from build123d import *

# Parameters (mm, degrees)
EXTRUDE_1_DEPTH          = 20
SKETCH_2_R               = 1.1
CUT_EXTRUDE_2_DEPTH      = 26.709920264
CUT_EXTRUDE_3_REACH      = 29.731
SKETCH_3_W               = 30
SKETCH_3_H               = 15.1
FILLET_1_R               = 3
SKETCH_6_W               = 30.918408881
SKETCH_6_H               = 20
SKETCH_6_W_2             = 27.918408881
SKETCH_6_H_2             = 17
EXTRUDE_2_DEPTH          = 2.5
CUT_EXTRUDE_4_DEPTH      = 25.9500604
CUT_EXTRUDE_4_DEPTH_BACK = 25.9500604


with BuildPart() as part:
    # 草图1 → 凸台-拉伸1 (new body)
    with BuildSketch(Plane(origin=(0, 0, 0), x_dir=(1, 0, 0), z_dir=(0, 1, 0))):
        Polygon((-15, -6), (15, 1.479840085), (15, 6), (-15, 6), align=None)
    extrude(amount=EXTRUDE_1_DEPTH)

    # 草图2 → 切除-拉伸2 (cut, through all)
    with BuildSketch(Plane(origin=(0, 20, 0), x_dir=(1, 0, 0), z_dir=(0, 1, 0))):
        with Locations(Location((-12.5, 3, 0), (0, 0, 270))):
            Circle(SKETCH_2_R)
        with Locations(Location((-7.537269242, 3.609346717, 0), (0, 0, 270))):
            Circle(SKETCH_2_R)
        with Locations(Location((-2.574538484, 4.218693434, 0), (0, 0, 270))):
            Circle(SKETCH_2_R)
    extrude(amount=-CUT_EXTRUDE_2_DEPTH, mode=Mode.SUBTRACT)

    # 切除-拉伸3: up to this plane
    cut_extrude_3_end = Plane(origin=(0.167638791, 0, 0.672362468), z_dir=(0.24192189559966876, 0, 0.9702957262759963))
    # 草图3 → 切除-拉伸3 (cut, up to the surface)
    with BuildSketch(Plane(origin=(0, 0, -6), x_dir=(-1, 0, 0), z_dir=(0, 0, -1)), mode=Mode.PRIVATE) as cut_extrude_3_sk1:
        with Locations((0, 10)):
            Rectangle(SKETCH_3_W, SKETCH_3_H)
    cut_extrude_3_tool1 = split(extrude(cut_extrude_3_sk1.sketch, amount=-CUT_EXTRUDE_3_REACH, mode=Mode.PRIVATE), bisect_by=cut_extrude_3_end, keep=Keep.BOTH, mode=Mode.PRIVATE)
    add(cut_extrude_3_tool1.solids().sort_by_distance((0, 10, -6))[0], mode=Mode.SUBTRACT)

    # 圆角1
    fillet_1_edges = [part.edges().sort_by_distance(p)[0] for p in [
        (-15, 1.225, -6),
        (-15, 18.775, -6),
    ]]
    fillet(fillet_1_edges, radius=FILLET_1_R)

    # 草图6 → 凸台-拉伸2 (add)
    with BuildSketch(Plane(origin=(0.530521635, 0, 2.127806058), x_dir=(0.9702957262759964, 0, -0.2419218955996687), z_dir=(0.2419218955996687, 0, 0.9702957262759964))):
        with Locations((-0.546762828, 10)):
            Rectangle(SKETCH_6_W, SKETCH_6_H)
        with Locations((-0.546762828, 10)):
            Rectangle(SKETCH_6_W_2, SKETCH_6_H_2, mode=Mode.SUBTRACT)
    extrude(amount=EXTRUDE_2_DEPTH)

    # 草图7 → 切除-拉伸4 (cut, two sides: drawn at the far end of the back side and taken through both)
    with BuildSketch(Plane(origin=(0, 2.45, 0), x_dir=(1, 0, 0), z_dir=(0, 1, 0)).offset(-CUT_EXTRUDE_4_DEPTH_BACK)):
        Polygon((15, 3.025760529), (4, 6), (15, 6), align=None)
    extrude(amount=CUT_EXTRUDE_4_DEPTH + CUT_EXTRUDE_4_DEPTH_BACK, mode=Mode.SUBTRACT)


solid = part.part
The listing builds one solid part. Answer for the finished solid, in the listing's coordinates (mm). A direction names the side the tool comes from. Coordinates: 2 decimals unless noted, no trailing zeros. Write each loop counter-clockwise with the first axis right and the second up, starting at its lowest first coordinate (ties: lowest second). Pieces come first, ordered by that corner, then holes. Notation, with made-up numbers: M 54,46 L 64,46 A20 cw 64,83 Z; hole C 83,28 d2. An arc over 180 degrees is marked long. Put each result on its own line as item: value. Start each with the question number.
1. A cutting plane is placed at B-B on x = -12.5. Write down the section's boundary in (y, z).
2. For a pull along Y with two mould halves and no side action, classify faces 1 (the flat face through (-0.21, 10.106, 0.767)), 2 (the flat face through (-1, 20, 0)), 3 (the flat face through (9.58, 1.21, -4.49)) as pulls with the +Y half, pulls with the -Y half, needs draft (parallel to the pull), parting line crosses it, or undercut.
3. Which of the six approach directions +Z, -Z, +X, -X, +Y, -Y give full straight-line access (tool end or side, diameter ignored) to faces 4 (the flat face through (15, 10, -2)), 5 (the flat face through (-4, 1, -6)), 6 (the flat face through (-3, 17.55, -2)), 7 (the cylindrical face through (-14.14, 1.24, -5.1)), 8 (the flat face through (13.843, 9.881, 0.079))?
4. A cutting plane is placed at D-D on x = 8. Write down the section's boundary in (y, z).
5. Consider line 1 (Y direction, x = 10.5, z = 0); line 2 (Y direction, x = -3, z = 0); line 3 (X direction, y = 18.4, z = -3). Determine where each line is inside the solid, lowest interval first. Write a range as from..to.
6. A cutting plane is placed at A-A on y = 15. Write down the section's boundary in (x, z).
7. Flat-ended cylindrical pins translate along their axes: P1, Ø1, axis at x = 0, y = 3.5, coming from the -Z side; P2, Ø10, axis at x = 6, y = 14.5, coming from the +Z side; P3, Ø2, axis at x = -12.5, z = -3, coming from the +Y side; P4, Ø6, axis at y = 10, z = -3, coming from the +X side. Find the tip coordinate at first contact, or state that the pin passes through.
8. A cutting plane is placed at C-C on z = 3.25. Write down the section's boundary in (x, y).
Resolved:
1. outline: M 0,-5.96 L 2.45,-5.96 L 2.45,-4.1 L 0,-4.1 Z; M 0,-1.9 L 2.45,-1.9 L 2.45,3.83 L 17.55,3.83 L 17.55,-1.9 L 20,-1.9 L 20,7.95 L 18.5,7.95 L 18.5,5.38 L 1.5,5.38 L 1.5,7.95 L 0,7.95 Z; M 17.55,-5.96 L 20,-5.96 L 20,-4.1 L 17.55,-4.1 Z
2. face 1: undercut
2. face 2: pulls with the +Y half
2. face 3: needs draft
3. face 4: -Z, +X, +Y, -Y
3. face 5: -Z, +X, -X, +Y, -Y
3. face 6: -Z, -X
3. face 7: -Z, -X, +Y, -Y
3. face 8: +Z
4. outline: M 0,-4.92 L 2.45,-4.92 L 2.45,-1.28 L 17.55,-1.28 L 17.55,-4.92 L 20,-4.92 L 20,2.84 L 18.5,2.84 L 18.5,0.27 L 1.5,0.27 L 1.5,2.84 L 0,2.84 Z
5. line 1: y = 0..1.5, 18.5..20
5. line 2: y = 0..2.45, 17.55..20
5. line 3: x = -15..-13.6, -11.4..-8.45, -6.62..15
6. outline: M -15,4.45 L 15,-3.03 L 15,-1.48 L 15.6,0.95 L 14.15,1.31 L 13.54,-1.12 L -13.54,5.64 L -12.94,8.06 L -14.4,8.43 L -15,6 Z
7. P1: stops at z = 0.59
7. P2: stops at z = 4.09
7. P3: passes through
7. P4: stops at x = 15.37
8. outline: M -15,0 L 6.36,0 L 6.36,1.5 L -3.97,1.5 L -3.97,18.5 L 6.36,18.5 L 6.36,20 L -15,20 L -15,17.55 L -10.17,17.55 L -10.17,2.45 L -15,2.45 Z
